from build123d import *

# Parameters (mm, degrees)
SKETCH1_R           = 7
BOSS_EXTRUDE1_DEPTH = 4.5
SKETCH3_R           = 2
CUT_EXTRUDE1_DEPTH  = 4
SKETCH4_R           = 2
CUT_EXTRUDE2_DEPTH  = 83.455425528
CUT_EXTRUDE3_DEPTH  = 83.769471168
CUT_EXTRUDE4_DEPTH  = 24
FILLET2_R           = 1
CUT_EXTRUDE5_DEPTH  = 1.264527456


# Read off the part's stored shape, not the designer's step: Cut-Extrude5
with BuildPart() as part:
    # Sketch1 → Boss-Extrude1 (new, symmetric)
    # profile 1 of 2: a face of its own
    with BuildSketch(Plane(origin=(0, 0, 0), x_dir=(1, 0, 0), z_dir=(0, 1, 0))):
        with BuildLine():
            ThreePointArc((-1.254341559, -11.934262744), (12, 0), (-1.254341559, 11.934262744))
            Line((-1.254341559, 11.934262744), (-30.046239367, 8.908112343))
            ThreePointArc((-30.046239367, 8.908112343), (-45.765521358, 9.327899994), (-60.835880843, 13.817478255))
            ThreePointArc((-60.835880843, 13.817478255), (-67.496359977, 15.745901742), (-74.430347821, 15.770640847))
            Line((-74.430347821, 15.770640847), (-69.554710794, 7.325789796))
            Line((-69.554710794, 7.325789796), (-62.626507563, 11.325789796))
            Line((-62.626507563, 11.325789796), (-56.626507563, 0.933484951))
            Line((-56.626507563, 0.933484951), (-63.554710794, -3.066515049))
            Line((-63.554710794, -3.066515049), (-60.930347821, -7.612045055))
            ThreePointArc((-60.930347821, -7.612045055), (-55.146607543, -6.760877199), (-49.301873665, -6.884263626))
            Line((-49.301873665, -6.884263626), (-1.254341559, -11.934262744))
        make_face()
        with Locations(Location((0, 0, 0), (0, 0, 270))):
            Circle(SKETCH1_R, mode=Mode.SUBTRACT)
    # profile 2 of 2: a face of its own
    with BuildSketch(Plane(origin=(0, 0, 0), x_dir=(1, 0, 0), z_dir=(0, 1, 0))):
        with BuildLine():
            Line((-69.554710794, 7.325789796), (-74.430347821, 15.770640847))
            ThreePointArc((-74.430347821, 15.770640847), (-81.705916239, 13.616086965), (-88, 9.37810303))
            Line((-88, 9.37810303), (-86.5, 6.780026819))
            Line((-86.5, 6.780026819), (-81.303847577, 9.780026819))
            Line((-81.303847577, 9.780026819), (-76.107695155, 6.780026819))
            Line((-76.107695155, 6.780026819), (-66.705771366, -9.504582872))
            ThreePointArc((-66.705771366, -9.504582872), (-63.859216184, -8.432717138), (-60.930347821, -7.612045055))
            Line((-60.930347821, -7.612045055), (-63.554710794, -3.066515049))
            Line((-63.554710794, -3.066515049), (-69.554710794, 7.325789796))
        make_face()
    extrude(amount=BOSS_EXTRUDE1_DEPTH, both=True)

    # Sketch3 → Cut-Extrude1 (cut)
    with BuildSketch(Plane(origin=(-20.560837732, 0, -35.612415597), x_dir=(0.8660254037844358, 0, -0.5000000000000051), z_dir=(0.500000000000005, 0, 0.8660254037844357))):
        with Locations((-52.573251602, 0)):
            Circle(SKETCH3_R)
    extrude(amount=-CUT_EXTRUDE1_DEPTH, mode=Mode.SUBTRACT)

    # Sketch4 → Cut-Extrude2 (cut, through all)
    with BuildSketch(Plane(origin=(-14.560837732, 0, -25.220110752), x_dir=(-0.8660254037844364, 0, 0.5000000000000041), z_dir=(-0.5000000000000041, 0, -0.8660254037844364))):
        with Locations(Location((52.573251602, 0, 0), (0, 0, 180))):
            Circle(SKETCH4_R)
    extrude(amount=-CUT_EXTRUDE2_DEPTH, mode=Mode.SUBTRACT)

    # Sketch6 → Cut-Extrude3 (cut, through all)
    with BuildSketch(Plane(origin=(-12.560837732, 0, -21.756009137), x_dir=(0.8660254037844358, 0, -0.5000000000000051), z_dir=(0.500000000000005, 0, 0.8660254037844357))):
        Polygon((-71.521184018, -2), (-62.521184018, -4.5), (-71.521184018, -4.5), align=None)
        Polygon((-62.521184018, 4.5), (-71.521184018, 4.5), (-71.521184018, 2), align=None)
    extrude(amount=-CUT_EXTRUDE3_DEPTH, mode=Mode.SUBTRACT)

    # Sketch6<4> → Cut-Extrude4 (cut)
    with BuildSketch(Plane(origin=(-12.560837732, 0, -21.756009137), x_dir=(0.8660254037844358, 0, -0.5000000000000051), z_dir=(0.500000000000005, 0, 0.8660254037844357))):
        with BuildLine():
            Line((-61.082433518, -1.25), (-65.521184018, -1.25))
            Line((-65.521184018, -1.25), (-65.521184018, 1.25))
            Line((-65.521184018, 1.25), (-61.082433518, 1.25))
            ThreePointArc((-61.082433518, 1.25), (-59.521184018, 2), (-57.959934518, 1.25))
            Line((-57.959934518, 1.25), (-56.521184018, 1.25))
            Line((-56.521184018, 1.25), (-56.521184018, -1.25))
            Line((-56.521184018, -1.25), (-57.959934518, -1.25))
            ThreePointArc((-57.959934518, -1.25), (-59.521184018, -2), (-61.082433518, -1.25))
        make_face()
    extrude(amount=-CUT_EXTRUDE4_DEPTH, mode=Mode.SUBTRACT)

    # Fillet2
    fillet2_edges = [part.edges().sort_by_distance(p)[0] for p in [
        (-56.626507563, 0, -0.933484951),
        (-62.626507563, 0, -11.325789796),
    ]]
    fillet(fillet2_edges, radius=FILLET2_R)

    # Cut-Extrude5 outline → Cut-Extrude5 (cut)
    with BuildSketch(Plane(origin=(-12.560837732, 0, -21.756009137), x_dir=(0.8660254037844358, 0, -0.5000000000000051), z_dir=(0.500000000000005, 0, 0.8660254037844357))):
        with BuildLine():
            ThreePointArc((-57.959934518, 1.25), (-59.521184018, 2), (-61.082433518, 1.25))
            Line((-61.082433518, 1.25), (-62.521184018, 1.25))
            Line((-62.521184018, 1.25), (-62.521184018, -1.25))
            Line((-62.521184018, -1.25), (-61.082433518, -1.25))
            ThreePointArc((-61.082433518, -1.25), (-59.521184018, -2), (-57.959934518, -1.25))
            Line((-57.959934518, -1.25), (-56.521184018, -1.25))
            Line((-56.521184018, -1.25), (-56.521184018, 1.25))
            Line((-56.521184018, 1.25), (-57.959934518, 1.25))
        make_face()
    extrude(amount=CUT_EXTRUDE5_DEPTH, mode=Mode.SUBTRACT)


solid = part.part
Source: CAD feature listing. Evaluate the final solid. Frame: model axes, mm. A direction names the side the tool comes from. Round coordinates to 2 decimals unless told otherwise and drop trailing zeros. Write each loop counter-clockwise with the first axis right and the second up, starting at its lowest first coordinate (ties: lowest second). Pieces come first, ordered by that corner, then holes. Notation, with made-up numbers: M 58,-0.75 L 95,-0.75 A11 ccw 95,9.25 Z; hole C 37.5,-2.5 d5. An arc over 180 degrees is marked long. One line per item, written item: value. Start each with the question number.
Item 1: Pin query (flat end, axial travel): pin 1 (1.5 mm diameter, centred on x = -3.5, y = 2.5, fed in from +Z); pin 2 (2 mm diameter, centred on y = 1, z = -11, fed in from +X); pin 3 (1.5 mm diameter, centred on x = -49, y = -2.5, fed in from -Z). Return the tip coordinate at first contact, or that it passes through.
Item 2: Section query A-A (x = 0). Return the cut outline in (y, z).
Item 3: Section query C-C (x = -41.5). Return the cut outline in (y, z).
Item 4: Section query B-B (z = -4.5). State how many separate pieces and enclosed holes the cut face has, plus the area to 3 significant figures.
Item 5: Mould query, pull axis Y, two halves, no side actions, for faces 1 (the flat face through (-68, 1.25, -3)), 2 (the flat face through (-68.11, 0.03, -12.78)), 3 (the flat face through (-82.34, 3.51, -10.45)), 4 (the cylindrical face through (12, 0, 0)). Classes: pulls with the +Y half, pulls with the -Y half, needs draft (parallel to the pull), parting line crosses it, or undercut.
Item 6: Ray query, L1, parallel to X at y = 2.5, z = -3.5; L2, parallel to Y at x = -66.5, z = -0.25; L3, parallel to X at y = -3.5, z = -4. Return the intervals inside material, ascending. Write a range as from..to.
Item 7: Set-up query: faces 5 (the cylindrical face through (-69.8, -2, -1.9)), 6 (the flat face through (-15.449, 0.063, -10.442)), 7 (the flat face through (-67.913, 1.063, -8.274)), 8 (the flat face through (-78.74, 2.54, -8.3)), 9 (the flat face through (-71.5, 0, -10.8)). Return all of +Z, -Z, +X, -X, +Y, -Y with unobstructed straight access to the full face (end or side cutting, diameter ignored); none if empty.
Result set:
1. pin 1: stops at z = 11.78
1. pin 2: stops at x = 6.63
1. pin 3: stops at z = -10.1
2. outline: M -4.5,-12 L 4.5,-12 L 4.5,-7 L -4.5,-7 Z; M -4.5,7 L 4.5,7 L 4.5,12 L -4.5,12 Z
3. outline: M -4.5,-8.8 L 4.5,-8.8 L 4.5,7.7 L -4.5,7.7 Z
4. separate pieces: 4
4. enclosed holes: 0
4. area: 573 mm²
5. face 1: undercut
5. face 2: undercut
5. face 3: pulls with the +Y half
5. face 4: needs draft
6. L1: x = -74.21..-67.35, -58.11..-6.06, 6.06..11.48
6. L2: y = -4.5..-1.25, 1.25..4.5
6. L3: x = -74.5..-67.63, -58.4..-5.74, 5.74..11.31
7. face 5: none
7. face 6: -Z, +Y, -Y
7. face 7: +Y, -Y
7. face 8: +Z, +Y, -Y
7. face 9: +Z
